Here's how the part is built. I have some questions about the finished solid (model axes, mm). Coordinates: 2 decimals unless noted, no trailing zeros. Loops run counter-clockwise (first coordinate to the right, second up) from the corner with the lowest first, then second, coordinate; pieces in that order, holes last.
```python
from build123d import *

# Parameters (mm, degrees)
SKETCH1_R           = 51.1048
SKETCH1_R_2         = 49.53
BOSS_EXTRUDE1_DEPTH = 812.8
CUT_EXTRUDE1_DEPTH  = 101.6


with BuildPart() as part:
    # Sketch1 → Boss-Extrude1 (new body)
    with BuildSketch(Plane(origin=(0, 0, 0), x_dir=(1, 0, 0), z_dir=(0, 1, 0))):
        with Locations(Location((0, 0, 0), (0, 0, 270))):
            Circle(SKETCH1_R)
        with Locations(Location((0, 0, 0), (0, 0, 270))):
            Circle(SKETCH1_R_2, mode=Mode.SUBTRACT)
    extrude(amount=BOSS_EXTRUDE1_DEPTH)

    # Sketch2 → Cut-Extrude1 (cut)
    with BuildSketch(Plane(origin=(0, 101.6, 0), x_dir=(-1, 0, 0), z_dir=(0, -1, 0))):
        with BuildLine():
            Line((-1.14808, 51.727157019), (-1.14808, 48.633812989))
            ThreePointArc((-1.14808, 48.633812989), (0, 48.647362247), (1.14808, 48.633812989))
            Line((1.14808, 48.633812989), (1.14808, 51.727157019))
            ThreePointArc((1.14808, 51.727157019), (0, 51.739896221), (-1.14808, 51.727157019))
        make_face()
        with BuildLine():
            Line((51.727157019, 1.14808), (48.633812989, 1.14808))
            ThreePointArc((48.633812989, 1.14808), (48.647362247, 0), (48.633812989, -1.14808))
            Line((48.633812989, -1.14808), (51.727157019, -1.14808))
            ThreePointArc((51.727157019, -1.14808), (51.739896221, 0), (51.727157019, 1.14808))
        make_face()
        with BuildLine():
            Line((1.14808, -51.727157019), (1.14808, -48.633812989))
            ThreePointArc((1.14808, -48.633812989), (0, -48.647362247), (-1.14808, -48.633812989))
            Line((-1.14808, -48.633812989), (-1.14808, -51.727157019))
            ThreePointArc((-1.14808, -51.727157019), (0, -51.739896221), (1.14808, -51.727157019))
        make_face()
        with BuildLine():
            Line((-51.727157019, -1.14808), (-48.633812989, -1.14808))
            ThreePointArc((-48.633812989, -1.14808), (-48.647362247, 0), (-48.633812989, 1.14808))
            Line((-48.633812989, 1.14808), (-51.727157019, 1.14808))
            ThreePointArc((-51.727157019, 1.14808), (-51.739896221, 0), (-51.727157019, -1.14808))
        make_face()
    extrude(amount=-CUT_EXTRUDE1_DEPTH, mode=Mode.SUBTRACT)


solid = part.part
```
1. I want a section at C-C (y = 461). Please give me the cut outline in (x, z).
2. We'd pull the mould along Z, two halves only. Please class faces 1 (the cylindrical face through (15.35, 400.71, 48.745)), 2 (the flat face through (27, 0, -42)), 3 (the cylindrical face through (14.88, 400.71, 47.24)): +Z half, -Z half, draft (parallel to the pull), parting line (faces both ways), or undercut.
3. I want a section at B-B (x = -31). Please give me the cut outline in (y, z), then the cut area to 3 significant figures.
4. I need wall thicknesses on line 1 along Z through (x, y) = (0, 331); line 2 along Z through (x, y) = (-38, 246.5). Which ranges of each line are inside material? Lowest first, please.
5. For pin 1 (3 mm diameter, centred on x = 35, y = 675, fed in from +Z); pin 2 (5 mm diameter, centred on x = 26, y = 463.5, fed in from +Z); pin 3 (2 mm diameter, centred on y = 492.5, z = -15.5, fed in from -X), each with a flat end and sliding along its axis, tell me the tip position at first contact or that it passes through.
6. I want a section at A-A (z = 34). Please give me the cut outline in (x, y), then the cut area to 3 significant figures.
Response values:
1. outline: circle Ø102.21 at (0, 0); hole circle Ø99.06 at (0, 0)
2. face 1: parting line
2. face 2: draft
2. face 3: undercut
3. outline: (0, -40.63) - (812.8, -40.63) - (812.8, -38.63) - (0, -38.63) - close; (0, 38.63) - (812.8, 38.63) - (812.8, 40.63) - (0, 40.63) - close
3. area: 3,250 mm2
4. line 1: z = -51.1 to -49.53, 49.53 to 51.1
4. line 2: z = -34.17 to -31.77, 31.77 to 34.17
5. pin 1: stops at z = 38.59
5. pin 2: stops at z = 45.38
5. pin 3: stops at x = -49
6. outline: (-38.15, 0) - (-36.02, 0) - (-36.02, 812.8) - (-38.15, 812.8) - close; (36.02, 0) - (38.15, 0) - (38.15, 812.8) - (36.02, 812.8) - close
6. area: 3,470 mm2
